Source: CAD feature listing. Evaluate the final solid. Frame: model axes, mm. Face numbers are marked on the shaded views. Round coordinates to 2 decimals unless told otherwise and drop trailing zeros. Loops run counter-clockwise (first coordinate to the right, second up) from the corner with the lowest first, then second, coordinate; pieces in that order, holes last. Notation, with made-up numbers: M -6.75,72 L 47.25,72 A21 ccw 47.25,110 Z; hole C 5,28 d9. An arc over 180 degrees is marked long. Answer as a JSON object with one key per item and string values.
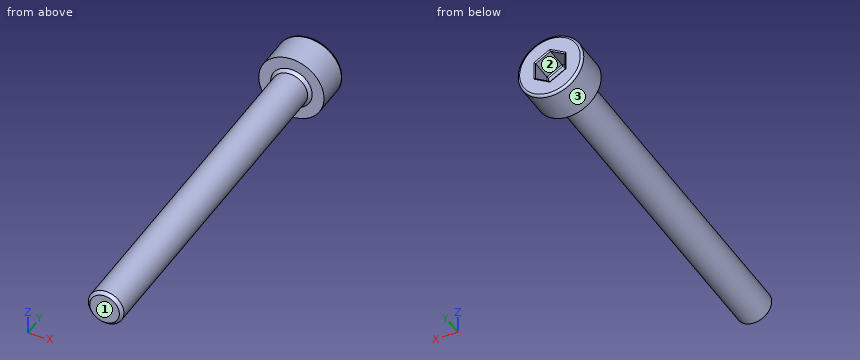
from build123d import *

# Parameters (mm, degrees)
CHAMFER1_SIZE      = 0.25
FILLET1_R          = 0.2
CUT_EXTRUDE1_DEPTH = 2
FILLET2_R          = 0.1


with BuildPart() as part:
    # Sketch1 → Revolve1 (revolve)
    with BuildSketch(Plane.XY):
        Polygon((0, -33), (-1.5, -33), (-1.5, -3), (-2.75, -3), (-2.75, 0), (0, 0), align=None)
    revolve(axis=Axis((0, 0, 0), (0, -1, 0)))

    # Chamfer1
    chamfer1_edges = [part.edges().sort_by_distance(p)[0] for p in [
        (1.5, -3, 0),
        (1.5, -33, 0),
    ]]
    chamfer(chamfer1_edges, length=CHAMFER1_SIZE)

    # Fillet1
    fillet1_edges = [part.edges().sort_by_distance(p)[0] for p in [
        (2.75, 0, 0),
    ]]
    fillet(fillet1_edges, radius=FILLET1_R)

    # Sketch2 → Cut-Extrude1 (cut)
    with BuildSketch(Plane(origin=(0, 0, 0), x_dir=(1, 0, 0), z_dir=(0, 1, 0))):
        Polygon((0, 1.443375673), (-1.25, 0.721687836), (-1.25, -0.721687836), (0, -1.443375673), (1.25, -0.721687836), (1.25, 0.721687836), align=None)
    extrude(amount=-CUT_EXTRUDE1_DEPTH, mode=Mode.SUBTRACT)

    # Fillet2
    fillet2_edges = [part.edges().sort_by_distance(p)[0] for p in [
        (0.625, -2, -1.082531755),
        (1.25, -2, 0),
        (0.625, -2, 1.082531755),
        (-0.625, -2, 1.082531755),
        (-1.25, -2, 0),
        (-0.625, -2, -1.082531755),
        (0.625, 0, -1.082531755),
        (-0.625, 0, -1.082531755),
        (-1.25, 0, 0),
        (-0.625, 0, 1.082531755),
        (0.625, 0, 1.082531755),
        (1.25, 0, 0),
    ]]
    fillet(fillet2_edges, radius=FILLET2_R)


solid = part.part
Item 1: Section B-B on y = -7. Return the cut outline in (x, z), then the cut area to 3 significant figures.
Answer sheet:
{"outline": "C 0,0 d3", "area": "7.07 mm²"}
Item 2: Section A-A on z = 0. Return the cut outline in (x, y), then the cut area to 3 significant figures.
Answer sheet:
{"outline": "M -2.75,-3 L -1.75,-3 L -1.5,-3.25 L -1.5,-32.75 L -1.25,-33 L 1.25,-33 L 1.5,-32.75 L 1.5,-3.25 L 1.75,-3 L 2.75,-3 L 2.75,-0.2 A0.2 ccw 2.55,0 L 1.35,0 A0.1 ccw 1.25,-0.1 L 1.25,-1.9 A0.1 cw 1.15,-2 L -1.15,-2 A0.1 cw -1.25,-1.9 L -1.25,-0.1 A0.1 ccw -1.35,0 L -2.55,0 A0.2 ccw -2.75,-0.2 Z", "area": "101 mm²"}
Item 3: Pull-direction query (X, two-part tool) for the marked faces 1, 2 and 3; classes: pulls with the +X half, pulls with the -X half, needs draft (parallel to the pull), parting line crosses it, or undercut.
Answer sheet:
{"face 1": "needs draft", "face 2": "undercut", "face 3": "parting line crosses it"}
Item 4: Contact query for flat-ended pins moving along their axis: pin 1 Ø2 at (x, y) = (0.5, -29) entering from +Z; pin 2 Ø2 at (x, y) = (-1.5, -21.5) entering from +Z; pin 3 Ø0.7 at (x, z) = (0.5, -0.5) entering from +Y. Output: stop coordinate, or through.
Answer sheet:
{"pin 1": "stops at z = 1.5", "pin 2": "stops at z = 1.41", "pin 3": "stops at y = -2"}
Item 5: Line query: probe 1 along Y at (x, z) = (0.45, 1.7); probe 2 along Z at (x, y) = (-0.7, -29); probe 3 along Y at (x, z) = (0.7, 0.25). Output: solid intervals per line, ascending. Write a range as from..to.
Answer sheet:
{"probe 1": "y = -3..0", "probe 2": "z = -1.33..1.33", "probe 3": "y = -33..-2"}
